Autodesk Inventor part; units mm, degrees
ref_plane "YZ Plane" through (0, 0, 0) normal (1, 0, 0) x (0, 1, 0)
ref_plane "XZ Plane" through (0, 0, 0) normal (0, 1, 0) x (-1, 0, 0)
ref_plane "XY Plane" through (0, 0, 0) normal (0, 0, 1) x (1, 0, 0)
sketch "Sketch1" plane through (0, 0, 0) normal (0, 0, 1) x (1, 0, 0)
  circle A0 centre (-2.6438, 6.9447) radius 6.8758
  line L0 (-9.4616, 7.8359) -> (-6.8245, 12.4034)
  line L1 (-6.8245, 1.4859) -> (-9.4616, 6.0534)
  line L2 (-0.0068, 0.5947) -> (-5.2808, 0.5947)
  line L3 (4.174, 6.0534) -> (1.537, 1.4859)
  line L4 (1.537, 12.4034) -> (4.174, 7.8359)
  line L5 (-5.2808, 13.2947) -> (-0.0068, 13.2947)
  point P0 (0, 0)
  point P1 (1.537, 1.4859)
  dimension "d0" = 13.7516
  dimension "d4" = 360
extrude "Extrusion1" add sketch "Sketch1" along normal blind 50.8 contours A0 L3 L2 L1 L0 L5 L4
sketch "Sketch2" plane through (0, 0, 50.8) normal (0, 0, 1) x (1, 0, 0)
  circle A0 centre (-2.6438, 6.9447) radius 2.5527
  line L0 (-5.2808, 0.5947) -> (-0.0068, 0.5947)
  line L1 (-2.6438, 6.9447) -> (-5.2808, 0.5947) construction
  line L2 (-2.6438, 6.9447) -> (-0.0068, 0.5947) construction
  point P0 (0, 0)
  dimension "d8" = 5.1054
  dimension "d9" = 6.35
extrude "Extrusion2" cut sketch "Sketch2" against normal blind 50.8
sketch "Sketch3" plane through (-5.2808, 13.2947, 0) normal (0, 1, 0) x (1, 0, 0)
  line L0 (0, 0) -> (5.274, 0)
  line L1 (1.6416, 0) -> (3.6416, 0)
  line L2 (3.6416, 0) -> (3.6416, -10)
  line L3 (3.6416, -10) -> (1.6416, -10)
  line L4 (1.6416, -10) -> (1.6416, 0)
  line L5 (2.6416, -10) -> (2.6416, 0) construction
  line L6 (0, 0) -> (0, -50.8)
  line L7 (5.274, 0) -> (5.274, -50.8)
  point P0 (5.2808, 0)
  dimension "d12" = 2
  dimension "d13" = 10
  dimension "d14" = 2.6416
extrude "Extrusion3" cut sketch "Sketch3" against normal blind 2
equation "\"d6\" = d5"
equation "\"d10\" = d5"
equation "\"d5\" = 50.8"
properties part number "Thundershaft 2in"
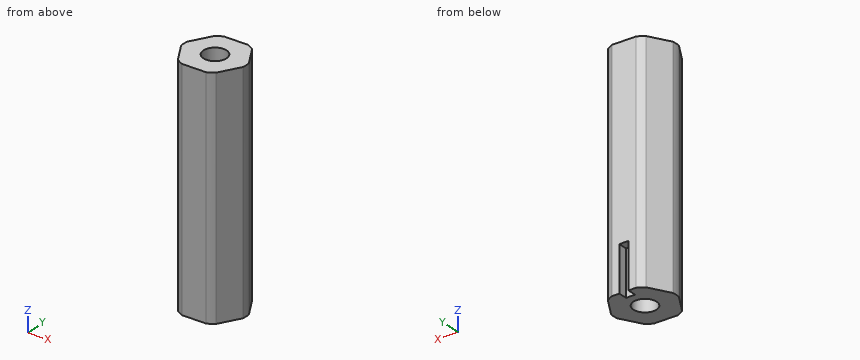
Check sheet for the modelled part. Datum: model origin and axes. Units: mm. Coordinates: 2 decimals unless noted, no trailing zeros. Loops run counter-clockwise (first coordinate to the right, second up) from the corner with the lowest first, then second, coordinate; pieces in that order, holes last.
1) Gauge pin test, flat ends, axial feed: pin 1 (0.6 mm diameter, centred on y = 12.5, z = 6, fed in from -X); pin 2 (1 mm diameter, centred on y = 12.5, z = 6.5, fed in from +X). Record the tip position at first contact, or that the pin passes through.
2) Material ranges on probe 1 along X at (y, z) = (5.25, 30); probe 2 along X at (y, z) = (6.5, 43); probe 3 along Y at (x, z) = (-1.25, 3.5), recorded low to high.
3) Sectioned sample at C-C (x = -8.5). Record the boundary of the cut face in (y, z), and give its area (3 significant figures).
4) Sectioned sample at A-A (y = 5). Record the boundary of the cut face in (x, z).
5) Sectioned sample at D-D (y = 2). Record the boundary of the cut face in (x, z), and give its area (3 significant figures).
6) Sectioned sample at B-B (z = 33.5). Record the boundary of the cut face in (x, y), and give its area (3 significant figures).
Check sheet entries:
1. pin 1: stops at x = -6.94
1. pin 2: stops at x = 1.77
2. probe 1: x = -9 to -4.55, -0.73 to 3.71
2. probe 2: x = -9.51 to -5.16, -0.13 to 4.22
2. probe 3: y = 0.59 to 4.81, 9.08 to 13.29
3. outline: (4.39, 0) - (9.5, 0) - (9.5, 50.8) - (4.39, 50.8) - close
3. area: 260 mm2
4. outline: (-8.85, 0) - (-4.3, 0) - (-4.3, 50.8) - (-8.85, 50.8) - close; (-0.99, 0) - (3.57, 0) - (3.57, 50.8) - (-0.99, 50.8) - close
5. outline: (-7.12, 0) - (1.83, 0) - (1.83, 50.8) - (-7.12, 50.8) - close
5. area: 455 mm2
6. outline: (-9.46, 6.05) - (-6.82, 1.49) arc R6.88 ccw to (-5.28, 0.59) - (-0.01, 0.59) arc R6.88 ccw to (1.54, 1.49) - (4.17, 6.05) arc R6.88 ccw to (4.17, 7.84) - (1.54, 12.4) arc R6.88 ccw to (-0.01, 13.29) - (-5.28, 13.29) arc R6.88 ccw to (-6.82, 12.4) - (-9.46, 7.84) arc R6.88 ccw to start; hole circle Ø5.11 at (-2.64, 6.94)
6. area: 117 mm2
